Build history of the part. All positions in model axes, mm. A direction names the side the tool comes from. Round coordinates to 2 decimals unless told otherwise and drop trailing zeros. Write each loop counter-clockwise with the first axis right and the second up, starting at its lowest first coordinate (ties: lowest second). Pieces come first, ordered by that corner, then holes.
from build123d import *

# Parameters (mm, degrees)
SKETCH1_R           = 23.5
BOSS_EXTRUDE1_DEPTH = 8
SKETCH2_R           = 38
BOSS_EXTRUDE2_DEPTH = 2
CUT_EXTRUDE1_START  = -2
SKETCH3_R           = 15
CUT_EXTRUDE1_DEPTH  = 53.332310829
SKETCH4_R           = 2
CUT_EXTRUDE2_DEPTH  = 55.332310829


with BuildPart() as part:
    # Sketch1 → Boss-Extrude1 (new body)
    with BuildSketch(Plane(origin=(0, 0, 0), x_dir=(1, 0, 0), z_dir=(0, 1, 0))):
        with Locations(Location((0, 0, 0), (0, 0, 270))):
            Circle(SKETCH1_R)
    extrude(amount=-BOSS_EXTRUDE1_DEPTH)

    # Sketch2 → Boss-Extrude2 (add)
    with BuildSketch(Plane(origin=(0, 0, 0), x_dir=(1, 0, 0), z_dir=(0, 1, 0))):
        with Locations(Location((0, 0, 0), (0, 0, 270))):
            Circle(SKETCH2_R)
    extrude(amount=-BOSS_EXTRUDE2_DEPTH)

    # Sketch3 → Cut-Extrude1 (cut, through all)
    with BuildSketch(Plane(origin=(0, 0, 0), x_dir=(1, 0, 0), z_dir=(0, 1, 0)).offset(CUT_EXTRUDE1_START)):
        with Locations(Location((0, 0, 0), (0, 0, 270))):
            Circle(SKETCH3_R)
    extrude(amount=-CUT_EXTRUDE1_DEPTH, mode=Mode.SUBTRACT)

    # Sketch4 → Cut-Extrude2 (cut, through all)
    with BuildSketch(Plane(origin=(0, 0, 0), x_dir=(1, 0, 0), z_dir=(0, 1, 0))):
        with Locations(Location((0, 31, 0), (0, 0, 270))):
            Circle(SKETCH4_R)
        with Locations(Location((31, 0, 0), (0, 0, 270))):
            Circle(SKETCH4_R)
        with Locations(Location((0, -31, 0), (0, 0, 270))):
            Circle(SKETCH4_R)
        with Locations(Location((-31, 0, 0), (0, 0, 270))):
            Circle(SKETCH4_R)
    extrude(amount=-CUT_EXTRUDE2_DEPTH, mode=Mode.SUBTRACT)


solid = part.part
1) Wall check: L1, parallel to X at y = -3.6, z = 0; L2, parallel to Y at x = 12.5, z = -5.5; L3, parallel to Z at x = 13.5, y = -4.25. Give the ranges that are in metal, low to high.
Results:
L1: x = -23.5 to -15, 15 to 23.5
L2: y = -2 to 0
L3: z = -19.24 to -6.54, 6.54 to 19.24
2) Slice it at A-A (z = 0). Write the cut outline in (x, y), plus the area to 3 significant figures.
Results:
outline: (-38, -2) - (-33, -2) - (-33, 0) - (-38, 0) - close; (-29, -2) - (-23.5, -2) - (-23.5, -8) - (-15, -8) - (-15, -2) - (15, -2) - (15, -8) - (23.5, -8) - (23.5, -2) - (29, -2) - (29, 0) - (-29, 0) - close; (33, -2) - (38, -2) - (38, 0) - (33, 0) - close
area: 238 mm2
3) Pin check, flat tips, straight feed: pin 1 Ø6.5 at (x, z) = (31, 0) entering from -Y; pin 2 Ø1.5 at (y, z) = (-2, 27) entering from -X. Stop position of each tip, or through.
Results:
pin 1: stops at y = -2
pin 2: stops at x = -27.48
4) Which spindle directions (+Z, -Z, +X, -X, +Y, -Y) get a long thin tool onto all of the face, cutting with end or side? Do faces 4 (the flat face through (0, -2, 0)), 5 (the cylindrical face through (-0.766, -0.986, 32.847)). Say none if no direction does.
Results:
face 4: -Y
face 5: +Y, -Y
5) Slice it at C-C (y = -1). Write the cut outline in (x, z).
Results:
outline: circle Ø76 at (0, 0); hole circle Ø4 at (-31, 0); hole circle Ø4 at (0, -31); hole circle Ø4 at (0, 31); hole circle Ø4 at (31, 0)
6) Slice it at D-D (z = 31). Write the cut outline in (x, y), plus the area to 3 significant figures.
Results:
outline: (-21.98, -2) - (-2, -2) - (-2, 0) - (-21.98, 0) - close; (2, -2) - (21.98, -2) - (21.98, 0) - (2, 0) - close
area: 79.9 mm2
7) Slice it at B-B (x = -31). Write the cut outline in (y, z).
Results:
outline: (-2, -21.98) - (0, -21.98) - (0, -2) - (-2, -2) - close; (-2, 2) - (0, 2) - (0, 21.98) - (-2, 21.98) - close
8) Mould opens along Z. For faces 1 (the cylindrical face through (-0.766, -0.986, -29.153)), 2 (the flat face through (17.4, -2, 16.4)), 3 (the cylindrical face through (-23.122, -0.986, -30.156)) say: released by +Z, released by -Z, zero draft, split by the parting line, or undercut.
Results:
face 1: undercut
face 2: zero draft
face 3: split by the parting line
